Check sheet for the modelled part. Datum: model origin and axes. Units: mm. A direction names the side the tool comes from. Round coordinates to 2 decimals unless told otherwise and drop trailing zeros. Loops run counter-clockwise (first coordinate to the right, second up) from the corner with the lowest first, then second, coordinate; pieces in that order, holes last. Notation, with made-up numbers: (74.25, -27) - (131.25, -27) arc R29 ccw to (131.25, 9) - close; hole circle Ø7 at (-19, -36.75). An arc over 180 degrees is marked (long way). Put each result on its own line as item: value.
Autodesk Inventor part; units mm, degrees
ref_plane "YZ Plane" through (0, 0, 0) normal (1, 0, 0) x (0, 1, 0)
ref_plane "XZ Plane" through (0, 0, 0) normal (0, 1, 0) x (-1, 0, 0)
ref_plane "XY Plane" through (0, 0, 0) normal (0, 0, 1) x (1, 0, 0)
sketch "Sketch1" plane through (0, 0, 0) normal (0, 1, 0) x (-1, 0, 0)
  line L0 (0, 0) -> (300, 0)
  line L1 (300, 0) -> (300, -100)
  line L2 (300, -100) -> (0, -100)
  line L3 (0, -100) -> (0, 0)
  dimension "d0" = 300
  dimension "d1" = 100
extrude "Extrusion1" add sketch "Sketch1" along normal blind 300
chamfer "Chamfer1" distance 250 distance2 250 1 edges at (-300, 0, -50) measured on face at (-100, 0, -33.3333)
shell "Shell1" thickness 2 removed faces 1 at (-100, 300, -33.3333)
sketch "Sketch2" plane through (0, 0, 0) normal (0, -1, 0) x (1, 0, 0)
  circle A0 centre (-26.2917, -50) radius 6.35
  point P0 (0, 0)
  dimension "d8" = 12.7
extrude "Extrusion2" add sketch "Sketch2" along normal blind 50
sketch "Sketch3" plane through (0, 0, 0) normal (1, 0, 0) x (0, 1, 0)
  circle A0 centre (-44.5235, -49.6457) radius 6.35
  point P0 (0, 0)
  dimension "d11" = 12.7
extrude "Extrusion3" add sketch "Sketch3" against normal blind 32 and the other way blind 200
fillet_without_effect "Fillet1"
sketch "Sketch4" plane through (0, 0, 0) normal (0, 0, 1) x (1, 0, 0)
  line L0 (-39.055, -25.4645) -> (218.0396, -25.4645)
  line L1 (218.0396, -25.4645) -> (218.0396, -67.5796)
  line L2 (218.0396, -67.5796) -> (-39.055, -67.5796)
  line L3 (-39.055, -67.5796) -> (-39.055, -25.4645)
  point P0 (0, 0)
extrude "Extrusion4" cut sketch "Sketch4" against normal blind 254
equation "\"BendRadius\" = Thickness"
equation "\"BendReliefWidth\" = Thickness"
equation "\"BendReliefDepth\" = 0.5 * Thickness"
equation "\"CornerReliefSize\" = 4 * Thickness"
equation "\"MinimumRemnant\" = 2 * Thickness"
equation "\"TransitionRadius\" = BendRadius"
equation "\"JacobiRadiusSize\" = Thickness"
equation "\"GapSize\" = Thickness"
properties part number "hopper 2"
Item 1: Section check A-A on z = -50. Enter the section's corners in (x, y).
Filled sheet:
outline: (-300, 250) - (-50, 0) - (-32.64, 0) - (-32.64, -25.46) - (-19.94, -25.46) - (-19.94, 0) - (0, 0) - (0, 300) - (-2, 300) - (-2, 2) - (-49.17, 2) - (-298, 250.83) - (-298, 300) - (-300, 300) - close
Item 2: Release check for a two-part mould opening along X. For faces 4 (the flat face through (-115, 182, -2)), 5 (the flat face through (-177, 127, -49)), 6 (the flat face through (-298, 275, -49)), 7 (the flat face through (-26, -25.464, -50)) record: +X half, -X half, draft (parallel to the pull), parting line (faces both ways), or undercut.
Filled sheet:
face 4: undercut
face 5: -X half
face 6: undercut
face 7: draft
Item 3: Section check D-D on z = -12. Enter the section's corners in (x, y), then the cut area to 3 significant figures.
Filled sheet:
outline: (-300, 250) - (-50, 0) - (0, 0) - (0, 300) - (-2, 300) - (-2, 2) - (-49.17, 2) - (-298, 250.83) - (-298, 300) - (-300, 300) - close
area: 1,500 mm²
Item 4: Thickness scan on line 1 (Z direction, x = -166, y = 246.5); line 2 (X direction, y = 275, z = -69); line 3 (X direction, y = 209, z = -15.5). Record the ranges inside material, lowest first. Write a range as from..to.
Filled sheet:
line 1: -100..-98, -2..0
line 2: -300..-298, -2..0
line 3: -259..-256.17, -2..0
Item 5: Tool access check on faces 1 (the flat face through (-175.33, 128.16, -49.33)), 2 (the flat face through (-115, 181, 0)), 3 (the cylindrical face through (-27.67, -12.55, -43.8)). Record the directions out of +Z, -Z, +X, -X, +Y, -Y that give a thin tool (end or side, any length) a straight path to the whole face; none if there is none.
Filled sheet:
face 1: +Y
face 2: +Z, +X, -X, +Y, -Y
face 3: -Y
Item 6: Section check C-C on x = -28. Enter the section's corners in (y, z), then the cut area to 3 significant figures.
Filled sheet:
outline: (-25.46, -56.12) - (0, -56.12) - (0, -100) - (300, -100) - (300, -98) - (2, -98) - (2, -2) - (300, -2) - (300, 0) - (0, 0) - (0, -43.88) - (-25.46, -43.88) - close
area: 1,700 mm²
Item 7: Section check B-B on y = 84.5. Enter the section's corners in (x, z), then the cut area to 3 significant figures.
Filled sheet:
outline: (-134.5, -100) - (0, -100) - (0, 0) - (-134.5, 0) - close; hole (-131.67, -98) - (-2, -98) - (-2, -2) - (-131.67, -2) - close
area: 1,000 mm²
Item 8: Go/stop test with flat-tipped pins: pin 1 (1.5 mm diameter, centred on y = 67, z = -85.5, fed in from +X); pin 2 (1.5 mm diameter, centred on x = -244.5, z = -80, fed in from +Y); pin 3 (4 mm diameter, centred on y = 234, z = -86, fed in from -X); pin 4 (1.5 mm diameter, centred on x = -236, z = -77.5, fed in from -Y). Record where each tip stops, or that it passes through.
Filled sheet:
pin 1: x = 0
pin 2: y = 198.08
pin 3: x = -286
pin 4: y = 185.25
